from build123d import *

# Parameters (mm, degrees)
SKETCH1_W           = 36
SKETCH1_H           = 128
BOSS_EXTRUDE1_DEPTH = 1
SKETCH2_W           = 36
SKETCH2_H           = 122
BOSS_EXTRUDE2_DEPTH = 6
SKETCH3_W           = 1
SKETCH3_H           = 6
BOSS_EXTRUDE3_DEPTH = 6
BOSS_EXTRUDE4_START = 3.5
BOSS_EXTRUDE4_DEPTH = 8


with BuildPart() as part:
    # Sketch1 → Boss-Extrude1 (new body)
    with BuildSketch(Plane(origin=(0, 0, 0), x_dir=(1, 0, 0), z_dir=(0, 1, 0))):
        Rectangle(SKETCH1_W, SKETCH1_H)
    extrude(amount=BOSS_EXTRUDE1_DEPTH)

    # Sketch2 → Boss-Extrude2 (add)
    with BuildSketch(Plane(origin=(0, 1, 0), x_dir=(1, 0, 0), z_dir=(0, 1, 0))):
        with Locations((0, -3)):
            Rectangle(SKETCH2_W, SKETCH2_H)
    extrude(amount=BOSS_EXTRUDE2_DEPTH)

    # Sketch3 → Boss-Extrude3 (add)
    with BuildSketch(Plane(origin=(0, 1, 0), x_dir=(1, 0, 0), z_dir=(0, 1, 0))):
        with Locations((-17.5, 61)):
            Rectangle(SKETCH3_W, SKETCH3_H)
    boss_extrude3 = extrude(amount=BOSS_EXTRUDE3_DEPTH)

    # Sketch4 → Boss-Extrude4 (add)
    with BuildSketch(Plane(origin=(0, 0, 0), x_dir=(0, 0, -1), z_dir=(1, 0, 0)).offset(BOSS_EXTRUDE4_START)):
        with BuildLine():
            Line((67.2, 1.2), (74, 1.2))
            Line((74, 1.2), (74, 1))
            Line((74, 1), (67.4, 1))
            ThreePointArc((67.4, 1), (67.258578644, 0.941421356), (67.2, 0.8))
            Line((67.2, 0.8), (67.2, 0.2))
            ThreePointArc((67.2, 0.2), (67.141421356, 0.058578644), (67, 0))
            Line((67, 0), (64, 0))
            Line((64, 0), (64, 0.2))
            Line((64, 0.2), (66.8, 0.2))
            ThreePointArc((66.8, 0.2), (66.941421356, 0.258578644), (67, 0.4))
            Line((67, 0.4), (67, 1))
            ThreePointArc((67, 1), (67.058578644, 1.141421356), (67.2, 1.2))
        make_face()
    boss_extrude4 = extrude(amount=BOSS_EXTRUDE4_DEPTH)

    # Mirror1: Boss-Extrude3, Boss-Extrude4 across plane
    add(boss_extrude3.mirror(Plane(origin=(0, 0, 0), x_dir=(0, 0, 1), z_dir=(1, 0, 0))))
    add(boss_extrude4.mirror(Plane(origin=(0, 0, 0), x_dir=(0, 0, 1), z_dir=(1, 0, 0))))


solid = part.part
Build history of the part. All positions in model axes, mm. A direction names the side the tool comes from. Coordinates: 2 decimals unless noted, no trailing zeros. Order: outer loops, then holes, each group sorted by start corner. A loop starts at its lowest first (then second) coordinate and runs counter-clockwise, first axis right, second up. Notation, with made-up numbers: (13.25, 40) - (46.25, 40) arc R8 ccw to (46.25, 49) - close; hole circle Ø4 at (19.5, -29.5). An arc over 180 degrees is marked (long way). Put each result on its own line as item: value.
1. Probe line 1 along Y through (x, z) = (-14, -59); line 2 along Z through (x, y) = (-8, 5.5). List the from-to ranges inside material, lowest first. Write a range as [from, to].
Answer sheet:
line 1: y = [0, 1]
line 2: z = [-58, 64]
2. Drop flat-ended pins along their axis: P1, Ø2, axis at x = 7, z = -70, coming from the +Y side; P2, Ø3, axis at x = 3, y = 4.5, coming from the -Z side; P3, Ø0.7, axis at x = -8.5, y = 0.5, coming from the -Z side. Give the stop position or say it passes through.
Answer sheet:
P1: stops at y = 1.2
P2: stops at z = -58
P3: stops at z = -67.21
3. Saw through at C-C (z = -61). Write the cut outline in (x, y), and give its area (3 significant figures).
Answer sheet:
outline: (-18, 0) - (18, 0) - (18, 7) - (17, 7) - (17, 1) - (-17, 1) - (-17, 7) - (-18, 7) - close
area: 48.0 mm^2
4. Saw through at A-A (x = 6). Write the cut outline in (y, z).
Answer sheet:
outline: (0, -67) arc R0.2 ccw to (0.2, -67.2) - (0.8, -67.2) arc R0.2 cw to (1, -67.4) - (1, -74) - (1.2, -74) - (1.2, -67.2) arc R0.2 ccw to (1, -67) - (0.4, -67) arc R0.2 cw to (0.2, -66.8) - (0.2, -64) - (1, -64) - (1, -58) - (7, -58) - (7, 64) - (0, 64) - close
5. Saw through at B-B (y = 4). Write the cut outline in (x, z).
Answer sheet:
outline: (-18, -64) - (-17, -64) - (-17, -58) - (17, -58) - (17, -64) - (18, -64) - (18, 64) - (-18, 64) - close
6. Tool access for faces 5 (the face through (7, 1, -71)), 6 (the face through (-7, 0.2, -65)), 7 (the face through (0, 1, -61)), 8 (the face through (-7, 1.2, -71)), 9 (the face through (17, 4, -61)): list every direction of +Z, -Z, +X, -X, +Y, -Y with a clear straight run to the whole face (end or side of a thin tool).
Answer sheet:
face 5: -Z, +X, -X, -Y
face 6: +X, -X, +Y
face 7: +Y
face 8: -Z, +X, -X, +Y
face 9: -Z, +Y
7. Pull direction X, two halves, no side cores. Call faces 1 (the face through (18, 3, 1)), 2 (the face through (-18, 3, 1)), 3 (the face through (-17, 4, -61)), 4 (the face through (7, 1.2, -71)): pulls with the +X half, pulls with the -X half, needs draft (parallel to the pull), parting line crosses it, or undercut.
Answer sheet:
face 1: pulls with the +X half
face 2: pulls with the -X half
face 3: undercut
face 4: needs draft
